Autodesk Inventor part; units mm, degrees
ref_plane "MSC_PF1" through (0, 0, 0) normal (1, 0, 0) x (0, 1, 0)
ref_plane "MSC_PT1" through (0, 0, 0) normal (0, 0, -1) x (-1, 0, 0)
ref_plane "YZ Plane" through (0, 0, 0) normal (1, 0, 0) x (0, 1, 0)
sketch "Esquisse1" plane through (0, 0, 0) normal (0, 1, 0) x (-1, 0, 0)
  point P0 (0, 0)
sketch "Esquisse2" plane through (0, 0, 0) normal (0, 0, 1) x (1, 0, 0)
  point P0 (0, 0)
sketch "Esquisse3" plane through (0, 0, 0) normal (0, 0, 1) x (1, 0, 0)
  point P0 (0, 0)
sketch "Esquisse4" plane through (0, 0, 0) normal (0, 1, 0) x (-1, 0, 0)
  line L0 (-2.75, 0) -> (0, 0)
  line L1 (-2.75, -0.4) -> (-2.75, 0)
  line L2 (-1.5, -1.65) -> (-2.75, -0.4)
  line L3 (-1.5, -1.9) -> (-1.5, -1.65)
  line L4 (-1.25, -2.15) -> (-1.5, -1.9)
  line L5 (-1.5, -2.4) -> (-1.25, -2.15)
  line L6 (-1.5, -10) -> (-1.5, -2.4)
  line L7 (0, 0) -> (0, -10)
  line L8 (0, 3.3392) -> (0, -10.7) construction
  line L9 (0, 3.3392) -> (0, -10.7)
  line L10 (0, -13.5078) -> (0, 6.1471)
  line L11 (-1.5, -10) -> (0, -10)
  line L12 (0.55, 0) -> (-3.3, 0)
  dimension "d3" = 2.75
  dimension "d5" = 0.25
  dimension "d7" = 0.25
  dimension "d9" = 0.25
  dimension "d11" = 1.65
  dimension "d13" = 135
  dimension "d17" = 1.25
  dimension "d19" = 0
  dimension "d51" = 1.5
  dimension "d52" = 10
revolve "Révolution1" add sketch "Esquisse4" angle 360 about axis through (0, 0, 3.3392) along (0, 0, -1)
sketch "Esquisse5" plane through (0, 0, 0) normal (0, 1, 0) x (-1, 0, 0)
  line L0 (-1.6, 0) -> (0, 0)
  line L1 (-0.2667, -1.5) -> (-1.6, 0)
  line L2 (0, -1.5) -> (-0.2667, -1.5)
  line L3 (0, 0) -> (0, -1.5)
  line L4 (-1.5, -1.65) -> (1.5, -1.65) construction
  line L5 (-2.75, 0) -> (2.75, 0)
  line L6 (0, -1.98) -> (0, 0.33)
  dimension "d22" = 1.6
  dimension "d24" = 0.2667
  dimension "d26" = 1.5
extrude "Extrusion1" cut sketch "Esquisse5" along normal mid plane 0.5333
pattern_circular "RéseauPolaire1" count 4 over 360 about axis through (0, 0, 0) along (0, 0, 1) of "Extrusion1"
sketch "Esquisse7" plane through (0, 0, 0) normal (0, 1, 0) x (-1, 0, 0)
  line L0 (0, -0.825) -> (-2, 0)
  line L1 (0, 0) -> (0, -0.825)
  line L2 (-2, 0) -> (0, 0)
  line L3 (-1.5, -1.65) -> (1.5, -1.65) construction
  line L4 (0, -1.98) -> (0, 0.33)
  line L5 (-2.75, 0) -> (2.75, 0)
  dimension "d33" = 2
  dimension "d35" = 0.825
extrude "Extrusion2" cut sketch "Esquisse7" along normal mid plane 0.5333
pattern_circular "RéseauPolaire2" count 4 over 360 about axis through (0, 0, 0) along (0, 0, 1) of "Extrusion2"
fillet "Congé1" radius 0.5 1 edges at (-1.5, 0, -1.65)
thread "Filetage1"
ref_plane "MSC_PF1" through (0, 0, 0) normal (1, 0, 0) x (0, 1, 0)
ref_plane "MSC_PT1" through (0, 0, 0) normal (0, 0, -1) x (-1, 0, 0)
equation "\"d3\" = 0.5 * Dh"
equation "\"d5\" = msp_x"
equation "\"d7\" = ParA"
equation "\"d9\" = msp_x"
equation "\"d11\" = ParK"
equation "\"d17\" = 0.5 * msp_mdtds"
equation "\"d51\" = 0.5 * NND"
equation "\"d52\" = NLG"
equation "\"d22\" = 0.5 * M"
equation "\"d24\" = 0.0833333 * M"
equation "\"d26\" = 0.909091 * ParK"
equation "\"d27\" = 0.166667 * M"
equation "\"d33\" = 0.625 * M"
equation "\"d35\" = 0.5 * ParK"
equation "\"d36\" = 0.166667 * M"
equation "\"d41\" = 2 * msp_x"
equation "\"PTC\" = 0.5"
equation "\"NLG\" = 10"
equation "\"ParK\" = 1.65"
equation "\"NND\" = 3"
equation "\"M\" = 3.2"
equation "\"msp_mdtds\" = NND - PTC"
equation "\"Dh\" = 5.5"
equation "\"msp_x\" = 0.5 * PTC"
equation "\"ParA\" = 0.5 * PTC"
equation "\"r\" = 0.8"
equation "\"THREADDIA\" = NND"
equation "\"TEMPLATE\" = 1.2345"
properties part number "NF EN ISO 7046-2 H - M3x10 - 8.8 - H1" material "Acier inoxydable 440C"
Work out the finished part from the listing and answer in its coordinate system (mm). A direction names the side the tool comes from. Round coordinates to 2 decimals unless told otherwise and drop trailing zeros. Write each loop counter-clockwise with the first axis right and the second up, starting at its lowest first coordinate (ties: lowest second). Pieces come first, ordered by that corner, then holes. Notation, with made-up numbers: (7.25, -8.75) - (60.25, -8.75) arc R32 ccw to (60.25, 18.25) - close; hole circle Ø11 at (-22.5, 49.25). An arc over 180 degrees is marked (long way). Return JSON: item names as keys, results as strings. Group by question number.
Q1. Find the intervals of material crossed by L1, parallel to Z at x = 1.1, y = -0.8; L2, parallel to Y at x = -0.7, z = -0.5; L3, parallel to X at y = -0.1, z = -7.75, in increasing order.
Q2. For faces 5 (the flat face through (0, -0.8, -0.9)), 6 (the flat face through (1, 1, 0)), determine the directions among +Z, -Z, +X, -X, +Y, -Y from which every point of the face is accessible in a straight line to the end or side of a thin tool.
Q3. The mould has two halves that part along X. Classify faces 1 (the cylindrical face through (-1.5, 0.07, -6.15)), 2 (the flat face through (0, 0, -10)), 3 (the flat face through (0.8, 0.267, -0.4)), 4 (the flat face through (0, 0.8, -0.9)): released by +X, released by -X, zero draft, split by the parting line, or undercut.
Q4. Each of these flat-tipped pins is pushed along its axis until it touches: pin 1 Ø0.8 at (y, z) = (-1, -1) entering from -X; pin 2 Ø0.6 at (x, y) = (0, 0) entering from +Z; pin 3 Ø1.2 at (x, z) = (-1.5, -1) entering from -Y. Where does it stop, or does it pass through?
Q5. The part is cut by section A-A on z = -9.5. Write down the section's boundary in (x, y), then the cut area to 3 significant figures.
Solved:
{
 "1": {"L1": "-10 to -2.26, -2.04 to 0", "L2": "-2.56 to -0.27, 0.27 to 2.56", "L3": "-1.5 to 1.5"},
 "2": {"face 5": "+Z", "face 6": "+Z, +X, -X, +Y, -Y"},
 "3": {"face 1": "split by the parting line", "face 2": "zero draft", "face 3": "undercut", "face 4": "undercut"},
 "4": {"pin 1": "x = -2.37", "pin 2": "z = -1.46", "pin 3": "y = -2.39"},
 "5": {"outline": "circle Ø3 at (0, 0)", "area": "7.07 mm²"}
}
